Source: CAD feature listing. Evaluate the final solid. Frame: model axes, mm. A direction names the side the tool comes from. Coordinates: 2 decimals unless noted, no trailing zeros. Write each loop counter-clockwise with the first axis right and the second up, starting at its lowest first coordinate (ties: lowest second). Pieces come first, ordered by that corner, then holes. Notation, with made-up numbers: M -19,29 L 1,29 A25 cw 1,59 Z; hole C 6.25,-31.75 d6. An arc over 180 degrees is marked long. One line per item, written item: value. Start each with the question number.
Item 1: Ray query, L1, parallel to X at y = 5, z = 11.75; L2, parallel to Y at x = 1.15, z = 12; L3, parallel to Z at x = 9.5, y = 35.5. Return the intervals inside material, ascending. Write a range as from..to.
Item 2: Pin query (flat end, axial travel): P1, Ø2.5, axis at y = 30.5, z = 12, coming from the -X side; P2, Ø0.8, axis at x = 23.5, z = 7.5, coming from the -Y side; P3, Ø2, axis at x = 34, y = 1.5, coming from the +Z side. Return the tip coordinate at first contact, or that it passes through.
Item 3: Cut plane D-D, the plane x = 20. Output: boundary loops of the cut face in (y, z).
Item 4: Cut plane B-B, the plane x = 45. Output: boundary loops of the cut face in (y, z), then the cut area to 3 significant figures.
Item 5: Mould query, pull axis Y, two halves, no side actions, for faces 1 (the cylindrical face through (1, 2, 15)), 2 (the flat face through (2, 18, 8)), 3 (the cylindrical face through (1, 36, 14)), 4 (the flat face through (102, 18, 8)). Classes: released by +Y, released by -Y, zero draft, split by the parting line, or undercut.
Item 6: Cut plane A-A, the plane z = 3.75. Output: boundary loops of the cut face in (x, y), then the cut area to 3 significant figures.
Item 7: Set-up query: faces 5 (the flat face through (0, 19, 8)), 6 (the flat face through (51, 2, 4)), 7 (the flat face through (51, 36, 8)). Return all of +Z, -Z, +X, -X, +Y, -Y with unobstructed straight access to the full face (end or side cutting, diameter ignored); none if empty.
Item 8: Cut plane C-C, the plane y = 24.5. Output: boundary loops of the cut face in (x, z), then the cut area to 3 significant figures.
```python
from build123d import *

# Parameters (mm, degrees)
F0_W          = 104
F0_H          = 37
F0_W_2        = 100
F0_H_2        = 33
F1_DEPTH      = 8
F3_DEPTH      = 1
F5_DEPTH      = 8
F6_R          = 0.75
F7_DEPTH      = 10.7
F7_DEPTH_BACK = 110.5
F8_R          = 5


with BuildPart() as f1:
    # F0 (on Top) → F1 (new body)
    with BuildSketch(Plane.XY):
        with Locations((52, 18.5)):
            Rectangle(F0_W, F0_H)
        with Locations((52, 18.5)):
            Rectangle(F0_W_2, F0_H_2, mode=Mode.SUBTRACT)
    extrude(amount=F1_DEPTH)

    # F2 (on face) → F3 (cut)
    with BuildSketch(Plane.XY.offset(8)):
        Polygon((46, 0), (52, 0), (58, 0), (58, 1), (52, 1), (46, 1), align=None)
        Polygon((18, 0), (24, 0), (29.75, 0), (29.75, 1), (23.75, 1), (18, 1), align=None)
        Polygon((73.25, 0), (80, 0), (85.25, 0), (85.25, 1), (79.25, 1), (73.25, 1), align=None)
    extrude(amount=-F3_DEPTH, mode=Mode.SUBTRACT)

    # F4 (on face) → F5 (join)
    with BuildSketch(Plane.XY.offset(8)):
        Polygon((0, 37), (0, 0), (2, 0), (2, 2), (2, 35), (2, 37), align=None)
        Polygon((104, 37), (102, 37), (102, 35), (102, 2), (102, 0), (104, 0), align=None)
    extrude(amount=F5_DEPTH)

    # F6 (on face) → F7 (cut, two sides)
    with BuildSketch(Plane(origin=(102, 0, 0), x_dir=(0, -1, 0), z_dir=(-1, 0, 0))) as f7_sk:
        with Locations((-30.5038709193, 12)):
            Circle(F6_R)
        with Locations((-11.9723072276, 12)):
            Circle(F6_R)
    extrude(amount=-F7_DEPTH, mode=Mode.SUBTRACT)
    extrude(f7_sk.sketch, amount=F7_DEPTH_BACK, mode=Mode.SUBTRACT)

    # F8
    f8_edges = [f1.edges().sort_by_distance(p)[0] for p in [
        (1, 0, 16),
        (103, 0, 16),
        (103, 37, 16),
        (1, 37, 16),
    ]]
    fillet(f8_edges, radius=F8_R)


solid = f1.part
```
From the geometry:
1. L1: x = 0..2, 102..104
1. L2: y = 0.1..11.22, 12.72..29.75, 31.25..36.9
1. L3: z = 0..8
2. P1: stops at x = 0
2. P2: stops at y = 1
2. P3: stops at z = 8
3. outline: M 0,0 L 2,0 L 2,8 L 1,8 L 1,7 L 0,7 Z; M 35,0 L 37,0 L 37,8 L 35,8 Z
4. outline: M 0,0 L 2,0 L 2,8 L 0,8 Z; M 35,0 L 37,0 L 37,8 L 35,8 Z
4. area: 32.0 mm²
5. face 1: released by -Y
5. face 2: undercut
5. face 3: released by +Y
5. face 4: undercut
6. outline: M 0,0 L 104,0 L 104,37 L 0,37 Z; hole M 2,2 L 102,2 L 102,35 L 2,35 Z
6. area: 548 mm²
7. face 5: +Z, -Z, -X, +Y, -Y
7. face 6: +Z, -Z
7. face 7: +Z, +Y, -Y
8. outline: M 0,0 L 2,0 L 2,16 L 0,16 Z; M 102,0 L 104,0 L 104,16 L 102,16 Z
8. area: 64.0 mm²
